```python
from build123d import *

# Parameters (mm, degrees)
F0_R     = 9.6
F1_DEPTH = 11
F2_R     = 11.125
F3_DEPTH = 1
F4_R     = 9.4
F5_DEPTH = 12.001


with BuildPart() as f1:
    # F0 (on Top) → F1 (new body)
    with BuildSketch(Plane.XY):
        Circle(F0_R)
    extrude(amount=F1_DEPTH)

    # F2 (on face) → F3 (join)
    with BuildSketch(Plane.XY.offset(11)):
        Circle(F2_R)
    extrude(amount=F3_DEPTH)

    # F4 (on face) → F5 (cut, through all)
    with BuildSketch(Plane(origin=(0, 0, 0), x_dir=(1, 0, 0), z_dir=(0, 0, -1))):
        Circle(F4_R)
    extrude(amount=-F5_DEPTH, mode=Mode.SUBTRACT)


solid = f1.part
```
The listing builds one solid part. Answer for the finished solid, in the listing's coordinates (mm). A direction names the side the tool comes from. Give positions to 0.01 mm unless a question says otherwise; leave off trailing zeros. Loops run counter-clockwise (first coordinate to the right, second up) from the corner with the lowest first, then second, coordinate; pieces in that order, holes last. Notation, with made-up numbers: (86.25, 17.5) - (94.25, 17.5) arc R27 cw to (94.25, 40.5) - close; hole circle Ø8 at (12, 17). An arc over 180 degrees is marked (long way). Return JSON: item names as keys, results as strings. Group by question number.
1. Given pin 1 Ø4 at (x, z) = (7, 3) entering from -Y; pin 2 Ø2 at (x, z) = (-5, 4) entering from -Y; pin 3 Ø3 at (y, z) = (0.5, 3) entering from +X, each flat-ended and moving along its own axis, determine where each tip first touches the part or whether it passes through.
2. Determine the mould class of faces 1 (the cylindrical face through (-2.038, 9.176, 5.916)), 2 (the cylindrical face through (5.161, 8.095, 5.423)), 3 (the flat face through (-5, 8.3, 12)) for opening direction Y: pulls with the +Y half, pulls with the -Y half, needs draft (parallel to the pull), parting line crosses it, or undercut.
3. Find section C-C (z = 8). Write down the section's boundary in (x, y), then the cut area to 3 significant figures.
4. Find section A-A (x = 0). Write down the section's boundary in (y, z) (3 decimals), then the cut area to 3 significant figures.
5. Straight lines are drawn through the part: line 1 (Y direction, x = 0, z = 8.5); line 2 (X direction, y = -5.25, z = 3.25); line 3 (X direction, y = -7.5, z = 2.5). For each, find the intervals that lie inside material, in ascending order. Write a range as [from, to].
6. Which of the six approach directions +Z, -Z, +X, -X, +Y, -Y give full straight-line access (tool end or side, diameter ignored) to faces 4 (the flat face through (-10, 0, 11)), 5 (the cylindrical face through (-8.2, 7.52, 11.49))?
Verdict:
{
 "1": {"pin 1": "stops at y = -8.2", "pin 2": "stops at y = -8.73", "pin 3": "stops at x = 9.6"},
 "2": {"face 1": "undercut", "face 2": "parting line crosses it", "face 3": "needs draft"},
 "3": {"outline": "circle Ø19.2 at (0, 0); hole circle Ø18.8 at (0, 0)", "area": "11.9 mm^2"},
 "4": {"outline": "(-11.125, 11) - (-9.6, 11) - (-9.6, 0) - (-9.4, 0) - (-9.4, 12) - (-11.125, 12) - close; (9.4, 0) - (9.6, 0) - (9.6, 11) - (11.125, 11) - (11.125, 12) - (9.4, 12) - close", "area": "7.85 mm^2"},
 "5": {"line 1": "y = [-9.6, -9.4], [9.4, 9.6]", "line 2": "x = [-8.04, -7.8], [7.8, 8.04]", "line 3": "x = [-5.99, -5.67], [5.67, 5.99]"},
 "6": {"face 4": "-Z", "face 5": "+Z, -Z"}
}
